Geometry: see drawing. Coordinates: mm, zero at the bounding-box minimum. Coordinates: 2 decimals unless noted, no trailing zeros. Write each loop counter-clockwise with the first axis right and the second up, starting at its lowest first coordinate (ties: lowest second). Pieces come first, ordered by that corner, then holes. Notation, with made-up numbers: (30, 19.25) -> (53, 19.25) arc R33 ccw to (53, 47.25) -> close; hole circle Ø4 at (57, 31). An arc over 180 degrees is marked (long way). Use one line per item in the form item = value. Start each with the question number.
(1) Ray query, line 1 along Z through (x, y) = (19, 7.75); line 2 along Y through (x, z) = (48, 29.5); line 3 along Y through (x, z) = (25, 1). Return the intervals inside material, ascending.
(2) Cut plane D-D on x = 17.5. Return the cut outline in (y, z).
(3) Cut plane C-C on y = 7.62. Return the cut outline in (x, z).
(4) First-contact query: pin 1 (0.8 mm diameter, centred on y = 4.5, z = 0.5, fed in from -X); pin 2 (19 mm diameter, centred on x = 18.5, z = 26.5, fed in from +Y); pin 3 (0.8 mm diameter, centred on y = 8, z = 0.5, fed in from +X). Flat tips, straight axial feed; report the tip coordinate or a pass-through.
(5) Pull-direction query (Z, two-part tool) for the marked faces 1, 2, 3 and 4; classes: released by +Z, released by -Z, zero draft, split by the parting line, or undercut.
(6) Cut plane A-A on y = 4.25. Return the cut outline in (x, z).
(7) Cut plane B-B on x = 25.4. Return the cut outline in (y, z).
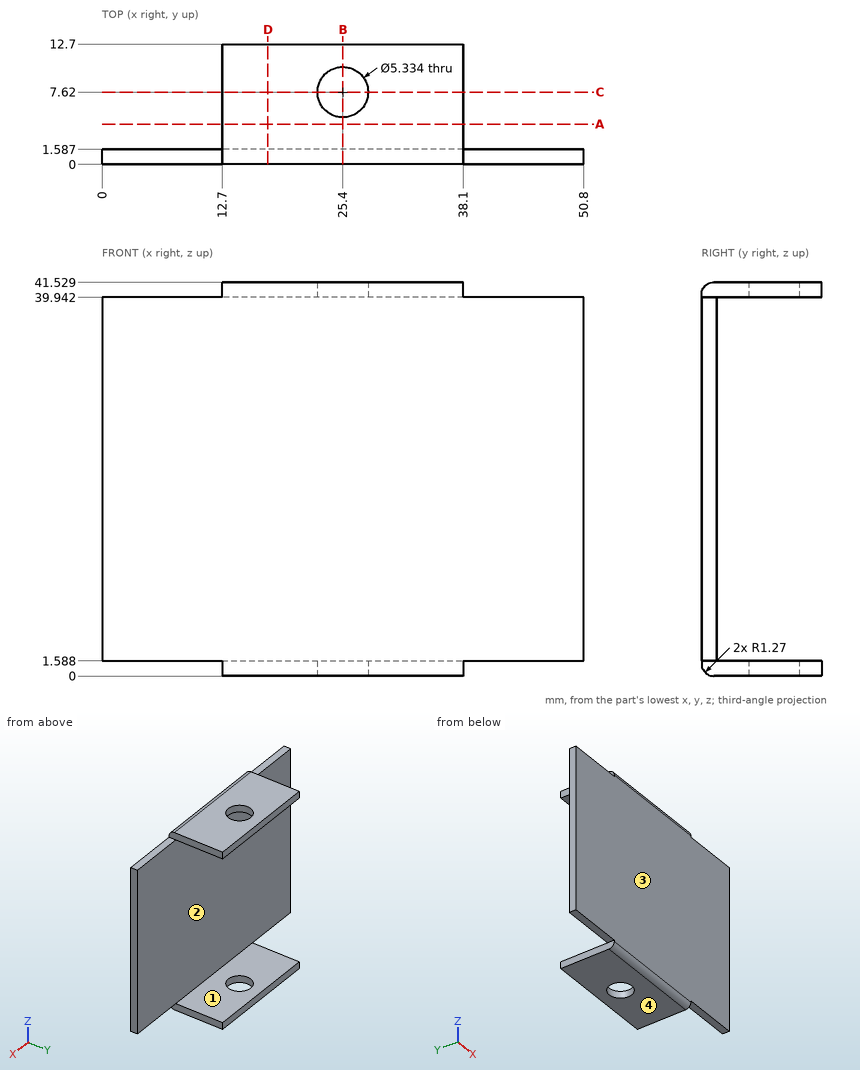
Values:
q1.line_1 = 0 to 1.59, 39.94 to 41.53
q1.line_2 = 0 to 1.59
q1.line_3 = 0.03 to 4.98, 10.26 to 12.7
q2.outline = (0, 1.27) arc R1.27 ccw to (1.27, 0) -> (12.7, 0) -> (12.7, 1.59) -> (1.59, 1.59) -> (1.59, 39.94) -> (12.7, 39.94) -> (12.7, 41.53) -> (1.27, 41.53) arc R1.27 ccw to (0, 40.26) -> close
q3.outline = (12.7, 0) -> (22.73, 0) -> (22.73, 1.59) -> (12.7, 1.59) -> close; (12.7, 39.94) -> (22.73, 39.94) -> (22.73, 41.53) -> (12.7, 41.53) -> close; (28.07, 0) -> (38.1, 0) -> (38.1, 1.59) -> (28.07, 1.59) -> close; (28.07, 39.94) -> (38.1, 39.94) -> (38.1, 41.53) -> (28.07, 41.53) -> close
q4.pin_1 = 12.7
q4.pin_2 = 1.59
q4.pin_3 = 38.1
q5.face_1 = undercut
q5.face_2 = undercut
q5.face_3 = zero draft
q5.face_4 = released by -Z
q6.outline = (12.7, 0) -> (38.1, 0) -> (38.1, 1.59) -> (12.7, 1.59) -> close; (12.7, 39.94) -> (38.1, 39.94) -> (38.1, 41.53) -> (12.7, 41.53) -> close
q7.outline = (0, 1.27) arc R1.27 ccw to (1.27, 0) -> (4.95, 0) -> (4.95, 1.59) -> (1.59, 1.59) -> (1.59, 39.94) -> (4.95, 39.94) -> (4.95, 41.53) -> (1.27, 41.53) arc R1.27 ccw to (0, 40.26) -> close; (10.29, 0) -> (12.7, 0) -> (12.7, 1.59) -> (10.29, 1.59) -> close; (10.29, 39.94) -> (12.7, 39.94) -> (12.7, 41.53) -> (10.29, 41.53) -> close
